Design review of the part built by this model. Coordinates are the model's own, in mm. A direction names the side the tool comes from. Give positions to 0.01 mm unless a question says otherwise; leave off trailing zeros. Order: outer loops, then holes, each group sorted by start corner. A loop starts at its lowest first (then second) coordinate and runs counter-clockwise, first axis right, second up.
Autodesk Inventor part; units mm, degrees
ref_plane "Work Plane1" through (0, 30, 0) normal (0, 1, 0) x (-1, 0, 0)
ref_plane "YZ Plane" through (0, 0, 0) normal (1, 0, 0) x (0, 1, 0)
ref_plane "XY Plane" through (0, 0, 0) normal (0, 0, 1) x (1, 0, 0)
sketch "Sketch1" plane through (0, 0, 0) normal (0, 0, 1) x (1, 0, 0)
  circle A0 centre (0, 0) radius 30
  dimension "d0" = 60
extrude "Extrusion1" add sketch "Sketch1" against normal blind 10
sketch "Sketch2" plane through (0, 0, -10) normal (0, 0, -1) x (-1, 0, 0)
  circle A0 centre (0, 0) radius 29
  dimension "d3" = 58
extrude "Extrusion2" cut sketch "Sketch2" against normal blind 8
ref_plane "Work Plane1" through (0, 30, 0) normal (0, 1, 0) x (-1, 0, 0)
sketch "Sketch3" plane through (0, 30, 0) normal (0, 1, 0) x (-1, 0, 0)
  line L0 (30, 0) -> (30, -10)
  line L1 (30, 0) -> (26, 0)
  line L2 (30, 0) -> (-30, 0)
  line L3 (26, 0) -> (24, 0)
  line L4 (24, 0) -> (24, -2)
  line L5 (24, -2) -> (26, -2)
  line L6 (26, -2) -> (26, 0)
  line L7 (24, 0) -> (21, 0)
  line L8 (21, 0) -> (19, 0)
  line L9 (19, 0) -> (19, -2)
  line L10 (19, -2) -> (21, -2)
  line L11 (21, -2) -> (21, 0)
  line L12 (19, 0) -> (16, 0)
  line L13 (16, 0) -> (14, 0)
  line L14 (14, 0) -> (14, -2)
  line L15 (14, -2) -> (16, -2)
  line L16 (16, -2) -> (16, 0)
  line L17 (14, 0) -> (11, 0)
  line L18 (11, 0) -> (9, 0)
  line L19 (9, 0) -> (9, -2)
  line L20 (9, -2) -> (11, -2)
  line L21 (11, -2) -> (11, 0)
  line L22 (9, 0) -> (6, 0)
  line L23 (6, 0) -> (4, 0)
  line L24 (4, 0) -> (4, -2)
  line L25 (4, -2) -> (6, -2)
  line L26 (6, -2) -> (6, 0)
  line L27 (4, 0) -> (1, 0)
  line L28 (1, 0) -> (-1, 0)
  line L29 (-1, 0) -> (-1, -2)
  line L30 (-1, -2) -> (1, -2)
  line L31 (1, -2) -> (1, 0)
  line L32 (-1, 0) -> (-4, 0)
  line L33 (-4, 0) -> (-6, 0)
  line L34 (-6, 0) -> (-6, -2)
  line L35 (-6, -2) -> (-4, -2)
  line L36 (-4, -2) -> (-4, 0)
  line L37 (-6, 0) -> (-9, 0)
  line L38 (-9, 0) -> (-11, 0)
  line L39 (-11, 0) -> (-11, -2)
  line L40 (-11, -2) -> (-9, -2)
  line L41 (-9, -2) -> (-9, 0)
  line L42 (-11, 0) -> (-14, 0)
  line L43 (-14, 0) -> (-16, 0)
  line L44 (-16, 0) -> (-16, -2)
  line L45 (-16, -2) -> (-14, -2)
  line L46 (-14, -2) -> (-14, 0)
  line L47 (-16, 0) -> (-19, 0)
  line L48 (-19, 0) -> (-21, 0)
  line L49 (-21, 0) -> (-21, -2)
  line L50 (-21, -2) -> (-19, -2)
  line L51 (-19, -2) -> (-19, 0)
  line L52 (-21, 0) -> (-24, 0)
  line L53 (-24, 0) -> (-26, 0)
  line L54 (-26, 0) -> (-26, -2)
  line L55 (-26, -2) -> (-24, -2)
  line L56 (-24, -2) -> (-24, 0)
  point P0 (0, 0)
  dimension "d7" = 4
  dimension "d8" = 2
  dimension "d9" = 2
  dimension "d10" = 3
  dimension "d11" = 2
  dimension "d12" = 2
  dimension "d13" = 3
  dimension "d14" = 2
  dimension "d15" = 2
  dimension "d16" = 3
  dimension "d17" = 2
  dimension "d18" = 2
  dimension "d19" = 3
  dimension "d20" = 2
  dimension "d21" = 2
  dimension "d22" = 3
  dimension "d23" = 2
  dimension "d24" = 2
  dimension "d25" = 3
  dimension "d26" = 2
  dimension "d27" = 2
  dimension "d28" = 3
  dimension "d29" = 2
  dimension "d30" = 2
  dimension "d31" = 3
  dimension "d32" = 2
  dimension "d33" = 2
  dimension "d34" = 3
  dimension "d35" = 2
  dimension "d36" = 2
  dimension "d37" = 3
  dimension "d38" = 2
  dimension "d39" = 2
extrude "Extrusion3" cut sketch "Sketch3" against normal through all
properties part number "fan front"
1. For line 1 along Y through (x, z) = (0, -7.25); line 2 along Y through (x, z) = (26, -4.75), list the stretches that pass through material, from the lowest coordinate up.
Recorded:
line 1: y = -30 to -29, 29 to 30
line 2: y = -14.97 to -12.85, 12.85 to 14.97
2. Machinability: for faces 3 (the face through (-8, 0, 0)), 4 (the face through (-10, -28, -2)), 5 (the face through (-17, 0, -2)), which of the approach directions +Z, -Z, +X, -X, +Y, -Y give a long, thin tool a straight path to every point of the face, cutting with its end or side? Answer none if there is none.
Recorded:
face 3: +Z, +X, -X, +Y, -Y
face 4: +Z, +Y, -Y
face 5: -Z
3. Take a section at A-A (x = 0). State the section outline as (y, z) points, then the cut area to 3 significant figures.
Recorded:
outline: (-30, -10) - (-29, -10) - (-29, -2) - (-30, -2) - close; (29, -10) - (30, -10) - (30, -2) - (29, -2) - close
area: 16.0 mm2
4. For pin 1 (12 mm diameter, centred on x = 6.5, y = 9, fed in from -Z); pin 2 (1 mm diameter, centred on x = 25, y = -16, fed in from +Z); pin 3 (1 mm diameter, centred on y = -7.5, z = -1, fed in from -X), all flat-tipped, find the tip position at first contact; note any pin that passes through.
Recorded:
pin 1: stops at z = -2
pin 2: stops at z = -2
pin 3: stops at x = -29.17
5. Take a section at C-C (y = 0). State how many separate pieces and enclosed holes the cut face has, then the cut area to 3 significant figures.
Recorded:
separate pieces: 12
enclosed holes: 0
area: 92.0 mm2
6. Draft analysis for pull direction Y (two halves, no side actions). For faces 1 (the face through (-13.38, -25.73, -6.06)), 2 (the face through (15, -25, -2)), state which applies: pulls with the +Y half, pulls with the -Y half, needs draft (parallel to the pull), parting line crosses it, or undercut.
Recorded:
face 1: undercut
face 2: needs draft
7. Take a section at B-B (z = -7.25). State the section outline as (x, y) points, then the cut area to 3 significant figures.
Recorded:
outline: circle Ø60 at (0, 0); hole circle Ø58 at (0, 0)
area: 185 mm2
8. Take a section at D-D (x = 15). State the section outline as (y, z) points, then the cut area to 3 significant figures.
Recorded:
outline: (-25.98, -10) - (-24.82, -10) - (-24.82, -2) - (-25.98, -2) - close; (24.82, -10) - (25.98, -10) - (25.98, -2) - (24.82, -2) - close
area: 18.6 mm2
